```python
from build123d import *

# Parameters (mm, degrees)
EXTRUDE1_DEPTH     = 3.3734375
SKETCH2_R          = 3.96875
CUT_EXTRUDE1_DEPTH = 11.269659873


with BuildPart() as part:
    # Sketch1 → Extrude1 (new body)
    with BuildSketch(Plane.XY):
        Polygon((0, 7.332348419), (-6.35, 3.666174209), (-6.35, -3.666174209), (0, -7.332348419), (6.35, -3.666174209), (6.35, 3.666174209), align=None)
    extrude1 = extrude(amount=EXTRUDE1_DEPTH)

    # Sketch2 → Cut-Extrude1 (cut, through all)
    with BuildSketch(Plane.XY.offset(3.3734375)):
        Circle(SKETCH2_R)
    cut_extrude1 = extrude(amount=-CUT_EXTRUDE1_DEPTH, mode=Mode.SUBTRACT)

    # Sketch3 → Cut-Revolve1 (revolve, cut)
    with BuildSketch(Plane(origin=(0, 0, 0), x_dir=(1, 0, 0), z_dir=(0, 1, 0))):
        Polygon((6.35, -3.3734375), (9.525, -0.709296171), (9.525, -3.3734375), align=None)
    cut_revolve1 = revolve(axis=Axis((0, 0, 0), (0, 0, 1)), mode=Mode.SUBTRACT)

    # Mirror1: Extrude1, Cut-Extrude1, Cut-Revolve1 across plane
    add(extrude1.mirror(Plane(origin=(0, 7.332348419, 0), x_dir=(1, 0, 0), z_dir=(0, 0, 1))))
    add(cut_extrude1.mirror(Plane(origin=(0, 7.332348419, 0), x_dir=(1, 0, 0), z_dir=(0, 0, 1))), mode=Mode.SUBTRACT)
    add(cut_revolve1.mirror(Plane(origin=(0, 7.332348419, 0), x_dir=(1, 0, 0), z_dir=(0, 0, 1))), mode=Mode.SUBTRACT)


solid = part.part
```
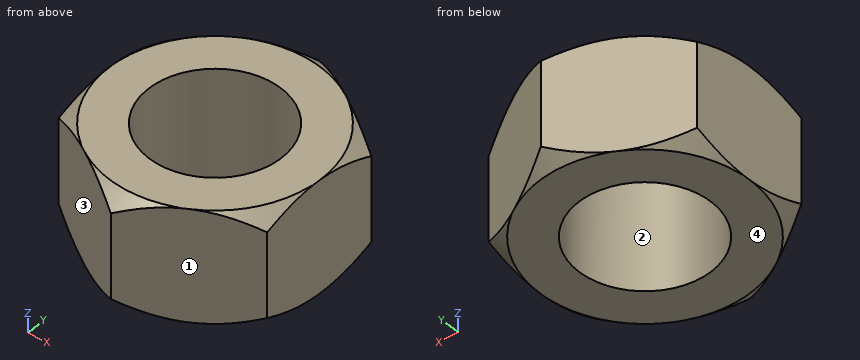
Part model, mm, in its own coordinate system. Face numbers are marked on the shaded views. Round coordinates to 2 decimals unless told otherwise and drop trailing zeros. Order: outer loops, then holes, each group sorted by start corner. A loop starts at its lowest first (then second) coordinate and runs counter-clockwise, first axis right, second up. Notation, with made-up numbers: M 53,52.5 L 96,52.5 A10 ccw 96,58.5 Z; hole C 41.5,86 d6. An arc over 180 degrees is marked long. Put each result on its own line as item: value. Start each with the question number.
1. Two-plate mould, pull along X, no slides. Class the marked faces 1, 2, 3 and 4: +X half, -X half, draft (parallel to the pull), parting line (faces both ways), or undercut.
2. Slice it at A-A on z = 0.25. List the corners of the cut face in (x, y).
3. Drop flat-ended pins along their axis: pin 1 (1 mm diameter, centred on x = -2.5, z = -0.5, fed in from +Y); pin 2 (6.5 mm diameter, centred on x = 0, y = 0, fed in from -Z); pin 3 (4 mm diameter, centred on x = 3, z = 0.5, fed in from +Y) (3 decimals); pin 4 (2 mm diameter, centred on x = -4, z = 0, fed in from -Y). Give the stop position or say it passes through.
4. Drill centre lines: probe 1 along X at (y, z) = (2.5, -2.25); probe 2 along Y at (x, z) = (2.5, -1.5); probe 3 along X at (y, z) = (-1.75, -1.5). Where is each one in solid material? Low to high. Write a range as [from, to].
Findings:
1. face 1: +X half
1. face 2: undercut
1. face 3: -X half
1. face 4: draft
2. outline: M -6.35,-3.67 L 0,-7.33 L 6.35,-3.67 L 6.35,3.67 L 0,7.33 L -6.35,3.67 Z; hole C 0,0 d7.94
3. pin 1: y = 6.18
3. pin 2: through
3. pin 3: y = 6.755
3. pin 4: y = -5.6
4. probe 1: [-6.35, -3.08], [3.08, 6.35]
4. probe 2: [-5.89, -3.08], [3.08, 5.89]
4. probe 3: [-6.35, -3.56], [3.56, 6.35]
